Geometry: final body of the model. Coordinates: model frame, mm. Face numbers are marked on the shaded views. Give positions to 0.01 mm unless a question says otherwise; leave off trailing zeros. Order: outer loops, then holes, each group sorted by start corner. A loop starts at its lowest first (then second) coordinate and runs counter-clockwise, first axis right, second up. Notation, with made-up numbers: M 61,53.5 L 115,53.5 A16 cw 115,67.5 Z; hole C 43.5,53.25 d3. An arc over 180 degrees is marked long. Write item = value, one per line. Start each with the question number.
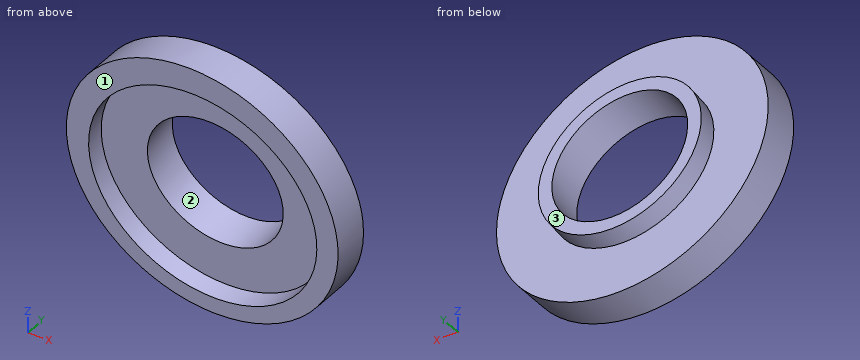
from build123d import *

# Parameters (mm, degrees)
SKETCH_1_R          = 25
EXTRUDE_1_DEPTH     = 30
CUT_EXTRUDE_1_DEPTH = 31.5
SKETCH_10_R         = 15
EXTRUDE_2_DEPTH     = 3.5
SKETCH_11_R         = 21
CUT_EXTRUDE_8_DEPTH = 3.5
SKETCH_12_R         = 12.5
CUT_EXTRUDE_9_DEPTH = 23.5


with BuildPart() as part:
    # 草图1 → 凸台-拉伸1 (new body)
    with BuildSketch(Plane(origin=(0, 0, 0), x_dir=(1, 0, 0), z_dir=(0, 1, 0))):
        Circle(SKETCH_1_R)
    extrude(amount=EXTRUDE_1_DEPTH)

    # 草图3 → 切除-拉伸1 (cut, symmetric)
    with BuildSketch(Plane(origin=(0, 0, 0), x_dir=(0, 0, -1), z_dir=(1, 0, 0))):
        Polygon((-25, 7), (25, 14.188898505), (25, 39.510034579), (-25, 39.510034579), align=None)
        Polygon((-25, 0), (25, 7.188898505), (25, -11.572478834), (-25, -11.572478834), align=None)
    extrude(amount=CUT_EXTRUDE_1_DEPTH, both=True, mode=Mode.SUBTRACT)

    # 草图10 → 凸台-拉伸2 (add)
    with BuildSketch(Plane(origin=(0, 10.379875382, 1.492397412), x_dir=(1, 0, 0), z_dir=(0, 0.989821487, 0.142314524))):
        with Locations((0, 1.507744004)):
            Circle(SKETCH_10_R)
    extrude(amount=EXTRUDE_2_DEPTH)

    # 草图11 → 切除-拉伸8 (cut)
    with BuildSketch(Plane(origin=(0, 3.521649349, 0.506335595), x_dir=(1, 0, 0), z_dir=(0, -0.989821487, -0.142314524))):
        with Locations((0, -1.507744004)):
            Circle(SKETCH_11_R)
    extrude(amount=-CUT_EXTRUDE_8_DEPTH, mode=Mode.SUBTRACT)

    # 草图12 → 切除-拉伸9 (cut)
    with BuildSketch(Plane(origin=(0, 13.844250587, 1.990498247), x_dir=(1, 0, 0), z_dir=(0, 0.989821487, 0.142314524))):
        with Locations((0, 1.507744004)):
            Circle(SKETCH_12_R)
    extrude(amount=-CUT_EXTRUDE_9_DEPTH, mode=Mode.SUBTRACT)


solid = part.part
1) Cut plane A-A (x = -9.5). Return loops of the section in (y, z) (3 decimals).
2) Cut plane B-B (x = 18). Return loops of the section in (y, z), plus the area to 3 significant figures.
3) Cut plane C-C (x = -4.5). Return loops of the section in (y, z), plus the area to 3 significant figures.
4) Ray query, L1, parallel to X at y = 9.25, z = -19; L2, parallel to X at y = 10.25, z = -9.5; L3, parallel to Y at x = -7.5, z = 16. Return the intervals inside material, ascending.
5) Draft query along Z for the marked faces 1, 2 and 3. Return one class per face: pulls with the +Z half, pulls with the -Z half, needs draft (parallel to the pull), parting line crosses it, or undercut.
6) Pin query (flat end, axial travel): pin 1 Ø1.5 at (x, y) = (-5.5, 10) entering from +Z; pin 2 Ø1 at (x, z) = (-0.5, 20) entering from +Y; pin 3 Ø8 at (y, z) = (9, 9) entering from -X. Return the tip coordinate at first contact, or that it passes through.
Reply:
q1.outline = M 0.27,23.125 L 1.071,17.552 L 4.535,18.05 L 6.044,7.553 L 12.903,8.539 L 12.407,11.988 L 8.942,11.49 L 7.27,23.125 Z; M 6.402,-19.524 L 6.919,-23.125 L 13.919,-23.125 L 12.246,-11.49 L 15.711,-10.992 L 15.215,-7.543 L 8.357,-8.529 L 9.866,-19.026 Z
q2.outline = M 1.1,17.35 L 2.2,9.72 L 5.66,10.22 L 8.74,-11.19 L 5.28,-11.69 L 6.09,-17.35 L 13.09,-17.35 L 8.1,17.35 Z
q2.area = 167 mm²
q3.outline = M 0.06,24.59 L 0.82,19.32 L 4.28,19.82 L 5.54,11.06 L 12.4,12.04 L 12.02,14.66 L 8.56,14.16 L 7.06,24.59 Z; M 6.66,-21.29 L 7.13,-24.59 L 14.13,-24.59 L 12.63,-14.16 L 16.1,-13.67 L 15.72,-11.05 L 8.86,-12.03 L 10.12,-20.79 Z
q3.area = 139 mm²
q4.L1 = -16.25 to -9.72, 9.72 to 16.25
q4.L2 = -23.12 to -8.29, 8.29 to 23.12
q4.L3 = 4.83 to 8.29
q5.face_1 = pulls with the -Z half
q5.face_2 = undercut
q5.face_3 = pulls with the +Z half
q6.pin_1 = 14.31
q6.pin_2 = 7.79
q6.pin_3 = -24.49
